Geometry: final body of the model. Coordinates: model frame, mm. Round coordinates to 2 decimals unless told otherwise and drop trailing zeros. Loops run counter-clockwise (first coordinate to the right, second up) from the corner with the lowest first, then second, coordinate; pieces in that order, holes last. Notation, with made-up numbers: (-31, 69) - (26, 69) arc R37 cw to (26, 108) - close; hole circle Ø2 at (69, -21.5). An arc over 180 degrees is marked (long way). Answer as a JSON object with one key per item and string values. Group by question number.
Item 1: Line query: line 1 (Z direction, x = 315, y = -11); line 2 (X direction, y = -14.25, z = 13.5); line 3 (Y direction, x = 399.5, z = 8). Output: solid intervals per line, ascending.
Item 2: Section A-A (x = 427). Return the cut outline in (y, z).
Item 3: First-contact query: pin 1 (14 mm diameter, centred on x = 683, z = 4, fed in from -Y); pin 2 (3 mm diameter, centred on y = -16.5, z = 51.5, fed in from +X); pin 3 (6.5 mm diameter, centred on x = 6, z = 116, fed in from -Y). Flat tips, straight axial feed; report the tip coordinate or a pass-through.
```python
from build123d import *

# Parameters (mm, degrees)
F0_W     = 965.2
F0_H     = 152.4
F1_DEPTH = 19.05
F2_W     = 12.7
F2_H     = 12.7
F3_DEPTH = 965.201
F4_W     = 12.7
F4_H     = 6.35
F5_DEPTH = 152.401
F6_W     = 12.7
F6_H     = 6.35
F7_DEPTH = 152.401


with BuildPart() as f1:
    # F0 (on Front) → F1 (new body)
    with BuildSketch(Plane.XZ):
        with Locations((482.6, 76.2)):
            Rectangle(F0_W, F0_H)
    extrude(amount=F1_DEPTH)

    # F2 (on face) → F3 (cut, through all)
    with BuildSketch(Plane(origin=(0, 0, 0), x_dir=(0, -1, 0), z_dir=(-1, 0, 0))):
        with Locations((12.7, 6.35)):
            Rectangle(F2_W, F2_H)
    extrude(amount=-F3_DEPTH, mode=Mode.SUBTRACT)

    # F4 (on face) → F5 (cut, through all)
    with BuildSketch(Plane(origin=(0, 0, 0), x_dir=(1, 0, 0), z_dir=(0, 0, -1))):
        with Locations((6.35, 15.875)):
            Rectangle(F4_W, F4_H)
    extrude(amount=-F5_DEPTH, mode=Mode.SUBTRACT)

    # F6 (on face) → F7 (cut, through all)
    with BuildSketch(Plane(origin=(0, 0, 0), x_dir=(1, 0, 0), z_dir=(0, 0, -1))):
        with Locations((958.85, 15.875)):
            Rectangle(F6_W, F6_H)
    extrude(amount=-F7_DEPTH, mode=Mode.SUBTRACT)


solid = f1.part
```
Values:
{
 "1": {"line 1": "z = 12.7 to 152.4", "line 2": "x = 12.7 to 952.5", "line 3": "y = -6.35 to 0"},
 "2": {"outline": "(-19.05, 12.7) - (-6.35, 12.7) - (-6.35, 0) - (0, 0) - (0, 152.4) - (-19.05, 152.4) - close"},
 "3": {"pin 1": "stops at y = -6.35", "pin 2": "stops at x = 952.5", "pin 3": "stops at y = -12.7"}
}
